Could you check a few things on this model? Use its own coordinates, in mm. A direction names the side the tool comes from. Give positions to 0.01 mm unless a question says otherwise; leave off trailing zeros. Write each loop counter-clockwise with the first axis right and the second up, starting at its lowest first coordinate (ties: lowest second). Pieces come first, ordered by that corner, then holes. Notation, with made-up numbers: M 28.25,9.25 L 72.25,9.25 A32 ccw 72.25,44.25 Z; hole C -33.75,70 d11. An arc over 180 degrees is marked long. Use one line per item in the form item = value.
from build123d import *

# Parameters (mm, degrees)
SKETCH1_W               = 50.8
SKETCH1_H               = 25.4
BOSS_EXTRUDE2_DEPTH     = 1066.8
CUT_EXTRUDE2_DEPTH      = 1069.310834917
CUT_EXTRUDE2_DEPTH_BACK = 1069.310834917
SKETCH3_W               = 44.45
SKETCH3_H               = 19.05
CUT_EXTRUDE3_DEPTH      = 1069.310834917
CUT_EXTRUDE3_DEPTH_BACK = 1069.310834917
SKETCH4_R               = 12.7


with BuildPart() as part:
    # Sketch1 → Boss-Extrude2 (new body)
    with BuildSketch(Plane.XY):
        with Locations((25.4, 12.7)):
            Rectangle(SKETCH1_W, SKETCH1_H)
    extrude(amount=BOSS_EXTRUDE2_DEPTH)

    # Sketch3 → Cut-Extrude2 (cut, two sides: drawn at the far end of the back side and taken through both)
    with BuildSketch(Plane.XY.offset(1066.8).offset(-CUT_EXTRUDE2_DEPTH_BACK)):
        with Locations((25.4, 12.7)):
            Rectangle(SKETCH3_W, SKETCH3_H)
    extrude(amount=CUT_EXTRUDE2_DEPTH + CUT_EXTRUDE2_DEPTH_BACK, mode=Mode.SUBTRACT)

    # Sketch4 → Cut-Extrude3 (cut, two sides: drawn at the far end of the back side and taken through both)
    with BuildSketch(Plane(origin=(0, 25.4, 0), x_dir=(1, 0, 0), z_dir=(0, 1, 0)).offset(-CUT_EXTRUDE3_DEPTH_BACK)):
        with Locations(Location((25.4, -1041.4, 0), (0, 0, 270))):
            Circle(SKETCH4_R)
    extrude(amount=CUT_EXTRUDE3_DEPTH + CUT_EXTRUDE3_DEPTH_BACK, mode=Mode.SUBTRACT)


solid = part.part
1) For faces 1 (the flat face through (3.175, 13, 526)), 2 (the flat face through (25, 25.4, 526)), which set-ups out of +Z, -Z, +X, -X, +Y, -Y let a thin tool reach every point of the face, with its end or its side?
Checked values:
face_1 = +Z, -Z
face_2 = +Z, -Z, +X, -X, +Y
2) I want a section at A-A, the plane z = 1041.4. Please give me the cut outline in (x, y) (3 decimals).
Checked values:
outline = M 0,0 L 12.7,0 L 12.7,3.175 L 3.175,3.175 L 3.175,22.225 L 12.7,22.225 L 12.7,25.4 L 0,25.4 Z; M 38.1,0 L 50.8,0 L 50.8,25.4 L 38.1,25.4 L 38.1,22.225 L 47.625,22.225 L 47.625,3.175 L 38.1,3.175 Z
3) Thinking about a two-plate mould opening in X: for faces 3 (the flat face through (50.8, 13, 526)), 4 (the flat face through (25, 23, 1066.8)), 5 (the flat face through (25, 22.225, 526)), which applies, released by +X, released by -X, zero draft, split by the parting line, or undercut?
Checked values:
face_3 = released by +X
face_4 = zero draft
face_5 = undercut
4) For pin 1 Ø12 at (x, z) = (37.5, 520) entering from -Y; pin 2 Ø5 at (x, y) = (22, 17.5) entering from +Z, each with a flat end and sliding along its axis, tell me the tip position at first contact or that it passes through.
Checked values:
pin_1 = 0
pin_2 = through
5) I want a section at C-C, the plane x = 25.4. Please give me the cut outline in (y, z) (3 decimals).
Checked values:
outline = M 0,0 L 3.175,0 L 3.175,1028.7 L 0,1028.7 Z; M 0,1054.1 L 3.175,1054.1 L 3.175,1066.8 L 0,1066.8 Z; M 22.225,0 L 25.4,0 L 25.4,1028.7 L 22.225,1028.7 Z; M 22.225,1054.1 L 25.4,1054.1 L 25.4,1066.8 L 22.225,1066.8 Z
6) I want a section at B-B, the plane y = 17.5. Please give me the cut outline in (x, z) (3 decimals).
Checked values:
outline = M 0,0 L 3.175,0 L 3.175,1066.8 L 0,1066.8 Z; M 47.625,0 L 50.8,0 L 50.8,1066.8 L 47.625,1066.8 Z
7) If I drill on L1, parallel to Z at x = 25.4, y = 24.6; L2, parallel to Y at x = 21, z = 44.5 (3 decimals); L3, parallel to X at y = 7.25, z = 938 (3 decimals), over which ranges is the centre line in solid material (lowest first)?
Checked values:
L1 = 0 to 1028.7, 1054.1 to 1066.8
L2 = 0 to 3.175, 22.225 to 25.4
L3 = 0 to 3.175, 47.625 to 50.8
